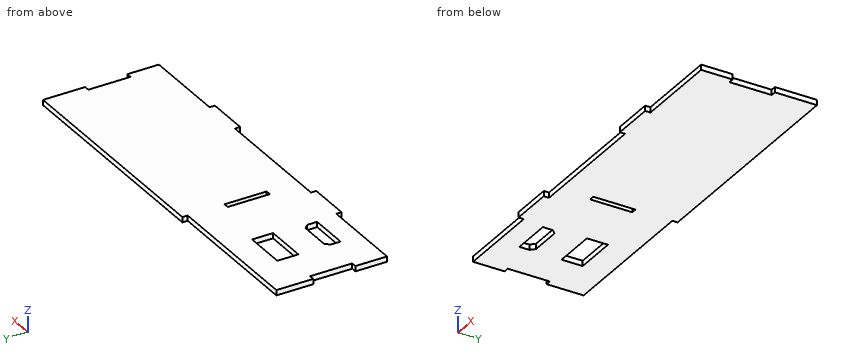
from build123d import *

# Parameters (mm, degrees)
SKETCH1_W           = 3.175
SKETCH1_H           = 25.4
BOSS_EXTRUDE1_DEPTH = 3.175
SKETCH2_W           = 25.4
SKETCH2_H           = 12.7
CUT_EXTRUDE1_DEPTH  = 4.175
SKETCH3_W           = 88.9
SKETCH3_H           = 3.175
CUT_EXTRUDE2_DEPTH  = 4.175


with BuildPart() as part:
    # Sketch1 → Boss-Extrude1 (new body)
    with BuildSketch(Plane.XY):
        Polygon((-114.3, 34.925), (-114.3, 9.525), (-111.125, 9.525), (-111.125, -15.875), (-114.3, -15.875), (-114.3, -34.925), (-63.5, -34.925), (-63.5, -38.1), (-38.1, -38.1), (-38.1, -34.925), (38.1, -34.925), (38.1, -38.1), (63.5, -38.1), (63.5, -34.925), (114.3, -34.925), (114.3, -15.875), (111.125, -15.875), (111.125, 9.525), (114.3, 9.525), (114.3, 34.925), align=None)
        with Locations((-26.9875, -3.175)):
            Rectangle(SKETCH1_W, SKETCH1_H, mode=Mode.SUBTRACT)
    extrude(amount=BOSS_EXTRUDE1_DEPTH)

    # Sketch2 → Cut-Extrude1 (cut, through all)
    with BuildSketch(Plane.XY.offset(3.175)):
        Polygon((-88.9, -16.225), (-86.4, -13.725), (-67.9, -13.725), (-65.4, -16.225), (-65.4, -22.225), (-88.9, -22.225), align=None)
        with Locations((-76.2, 9.525)):
            Rectangle(SKETCH2_W, SKETCH2_H)
    extrude(amount=-CUT_EXTRUDE1_DEPTH, mode=Mode.SUBTRACT)

    # Sketch3 → Cut-Extrude2 (cut, through all)
    with BuildSketch(Plane.XY.offset(3.175)):
        with Locations((-69.85, 33.3375)):
            Rectangle(SKETCH3_W, SKETCH3_H)
    extrude(amount=-CUT_EXTRUDE2_DEPTH, mode=Mode.SUBTRACT)


solid = part.part
Verification items for the finished model (mm, model axes). Give positions to 0.01 mm unless a question says otherwise; leave off trailing zeros. Order: outer loops, then holes, each group sorted by start corner. A loop starts at its lowest first (then second) coordinate and runs counter-clockwise, first axis right, second up. Notation, with made-up numbers: M 45.25,14 L 52.25,14 A12 cw 52.25,20 Z; hole C 29.5,61 d5. An arc over 180 degrees is marked long. Answer as a JSON object with one key per item and string values. Group by question number.
1) Scan lines: line 1 along Y through (x, z) = (-73, 2.8) (3 decimals); line 2 along X through (y, z) = (-5, 2.05) (3 decimals); line 3 along X through (y, z) = (-17.5, 1.75). Record each from-to range of solid material in increasing order. Write a range as [from, to].
2) Cross-section at D-D (x = 98). Enter the section's corners in (y, z) (3 decimals).
3) Cross-section at C-C (x = -36). Enter the section's corners in (y, z) (3 decimals), then the cut area to 3 significant figures.
4) Cross-section at A-A (x = -75.5). Enter the section's corners in (y, z) (3 decimals), then the cut area to 3 significant figures.
5) Depth check by flat-ended pin: pin 1 Ø1.6 at (y, z) = (-37, 1) entering from -X; pin 2 Ø1.6 at (y, z) = (-6.5, 2) entering from +X (3 decimals); pin 3 Ø1 at (x, z) = (-91.5, 1.5) entering from +Y. Enter the tip coordinate at first touch or a pass-through.
6) Cross-section at B-B (z = 0.75). Give the number of separate pieces and of enclosed holes in the cut face, then the cut area to 3 significant figures.
Result sheet:
{
 "1": {"line 1": "y = [-34.925, -22.225], [-13.725, 3.175], [15.875, 31.75]", "line 2": "x = [-111.125, -28.575], [-25.4, 111.125]", "line 3": "x = [-114.3, -88.9], [-65.4, 114.3]"},
 "2": {"outline": "M -34.925,0 L 34.925,0 L 34.925,3.175 L -34.925,3.175 Z"},
 "3": {"outline": "M -34.925,0 L 31.75,0 L 31.75,3.175 L -34.925,3.175 Z", "area": "212 mm2"},
 "4": {"outline": "M -34.925,0 L -22.225,0 L -22.225,3.175 L -34.925,3.175 Z; M -13.725,0 L 3.175,0 L 3.175,3.175 L -13.725,3.175 Z; M 15.875,0 L 31.75,0 L 31.75,3.175 L 15.875,3.175 Z", "area": "144 mm2"},
 "5": {"pin 1": "stops at x = -63.5", "pin 2": "stops at x = 111.125", "pin 3": "stops at y = 31.75"},
 "6": {"separate pieces": "1", "enclosed holes": "3", "area": "15,100 mm2"}
}
